Here's how the part is built. I have some questions about the finished solid (model axes, mm). Coordinates: 2 decimals unless noted, no trailing zeros. Order: outer loops, then holes, each group sorted by start corner. A loop starts at its lowest first (then second) coordinate and runs counter-clockwise, first axis right, second up.
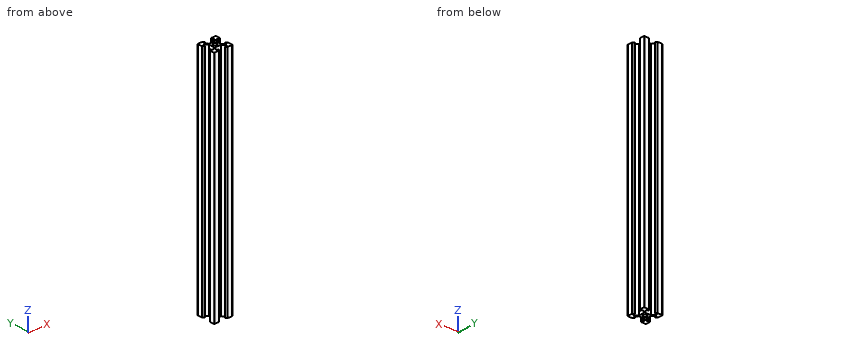
```python
from build123d import *

# Parameters (mm, degrees)
SKETCH1_R           = 2.05
BOSS_EXTRUDE1_DEPTH = 250


with BuildPart() as part:
    # Sketch1 → Boss-Extrude1 (new body)
    with BuildSketch(Plane(origin=(0, 0, 0), x_dir=(0, 1, 0), z_dir=(0, 0, 1))):
        with BuildLine():
            Line((-2.860050506, -3.85), (2.860050506, -3.85))
            Line((2.860050506, -3.85), (5.5, -6.489949494))
            Line((5.5, -6.489949494), (5.5, -8.1))
            Line((5.5, -8.1), (3.382842712, -8.1))
            ThreePointArc((3.382842712, -8.1), (3.198066806, -8.223463314), (3.241421356, -8.441421356))
            Line((3.241421356, -8.441421356), (4.624264069, -9.824264069))
            ThreePointArc((4.624264069, -9.824264069), (4.818918078, -9.95432772), (5.048528137, -10))
            Line((5.048528137, -10), (9.5, -10))
            ThreePointArc((9.5, -10), (9.853553391, -9.853553391), (10, -9.5))
            Line((10, -9.5), (10, -5.048528137))
            ThreePointArc((10, -5.048528137), (9.95432772, -4.818918078), (9.824264069, -4.624264069))
            Line((9.824264069, -4.624264069), (8.441421356, -3.241421356))
            ThreePointArc((8.441421356, -3.241421356), (8.223463314, -3.198066806), (8.1, -3.382842712))
            Line((8.1, -3.382842712), (8.1, -5.5))
            Line((8.1, -5.5), (6.489949494, -5.5))
            Line((6.489949494, -5.5), (3.85, -2.860050506))
            Line((3.85, -2.860050506), (3.85, 2.860050506))
            Line((3.85, 2.860050506), (6.489949494, 5.5))
            Line((6.489949494, 5.5), (8.1, 5.5))
            Line((8.1, 5.5), (8.1, 3.382842712))
            ThreePointArc((8.1, 3.382842712), (8.223463314, 3.198066806), (8.441421356, 3.241421356))
            Line((8.441421356, 3.241421356), (9.824264069, 4.624264069))
            ThreePointArc((9.824264069, 4.624264069), (9.95432772, 4.818918078), (10, 5.048528137))
            Line((10, 5.048528137), (10, 9.5))
            ThreePointArc((10, 9.5), (9.853553391, 9.853553391), (9.5, 10))
            Line((9.5, 10), (5.048528137, 10))
            ThreePointArc((5.048528137, 10), (4.818918078, 9.95432772), (4.624264069, 9.824264069))
            Line((4.624264069, 9.824264069), (3.241421356, 8.441421356))
            ThreePointArc((3.241421356, 8.441421356), (3.198066806, 8.223463314), (3.382842712, 8.1))
            Line((3.382842712, 8.1), (5.5, 8.1))
            Line((5.5, 8.1), (5.5, 6.489949494))
            Line((5.5, 6.489949494), (2.860050506, 3.85))
            Line((2.860050506, 3.85), (-2.860050506, 3.85))
            Line((-2.860050506, 3.85), (-5.5, 6.489949494))
            Line((-5.5, 6.489949494), (-5.5, 8.1))
            Line((-5.5, 8.1), (-3.382842712, 8.1))
            ThreePointArc((-3.382842712, 8.1), (-3.198066806, 8.223463314), (-3.241421356, 8.441421356))
            Line((-3.241421356, 8.441421356), (-4.624264069, 9.824264069))
            ThreePointArc((-4.624264069, 9.824264069), (-4.818918078, 9.95432772), (-5.048528137, 10))
            Line((-5.048528137, 10), (-9.5, 10))
            ThreePointArc((-9.5, 10), (-9.853553391, 9.853553391), (-10, 9.5))
            Line((-10, 9.5), (-10, 5.048528137))
            ThreePointArc((-10, 5.048528137), (-9.95432772, 4.818918078), (-9.824264069, 4.624264069))
            Line((-9.824264069, 4.624264069), (-8.441421356, 3.241421356))
            ThreePointArc((-8.441421356, 3.241421356), (-8.223463314, 3.198066806), (-8.1, 3.382842712))
            Line((-8.1, 3.382842712), (-8.1, 5.5))
            Line((-8.1, 5.5), (-6.489949494, 5.5))
            Line((-6.489949494, 5.5), (-3.85, 2.860050506))
            Line((-3.85, 2.860050506), (-3.85, -2.860050506))
            Line((-3.85, -2.860050506), (-6.489949494, -5.5))
            Line((-6.489949494, -5.5), (-8.1, -5.5))
            Line((-8.1, -5.5), (-8.1, -3.382842712))
            ThreePointArc((-8.1, -3.382842712), (-8.223463314, -3.198066806), (-8.441421356, -3.241421356))
            Line((-8.441421356, -3.241421356), (-9.824264069, -4.624264069))
            ThreePointArc((-9.824264069, -4.624264069), (-9.95432772, -4.818918078), (-10, -5.048528137))
            Line((-10, -5.048528137), (-10, -9.5))
            ThreePointArc((-10, -9.5), (-9.853553391, -9.853553391), (-9.5, -10))
            Line((-9.5, -10), (-5.048528137, -10))
            ThreePointArc((-5.048528137, -10), (-4.818918078, -9.95432772), (-4.624264069, -9.824264069))
            Line((-4.624264069, -9.824264069), (-3.241421356, -8.441421356))
            ThreePointArc((-3.241421356, -8.441421356), (-3.198066806, -8.223463314), (-3.382842712, -8.1))
            Line((-3.382842712, -8.1), (-5.5, -8.1))
            Line((-5.5, -8.1), (-5.5, -6.489949494))
            Line((-5.5, -6.489949494), (-2.860050506, -3.85))
        make_face()
        with Locations(Location((0, 0, 0), (0, 0, 270))):
            Circle(SKETCH1_R, mode=Mode.SUBTRACT)
    extrude(amount=BOSS_EXTRUDE1_DEPTH)


solid = part.part
```
Q1. Will these pins go through, and if not, where does the flat tip stop? pin 1 (8 mm diameter, centred on x = 1, z = 134.5, fed in from -Y); pin 2 (6.5 mm diameter, centred on y = 1.5, z = 129, fed in from -X); pin 3 (0.6 mm diameter, centred on y = 4, z = 113, fed in from -X); pin 4 (1.5 mm diameter, centred on x = -1, y = 6, fed in from +Z).
Q2. If we section it at A-A on x = 0: Write out the boundary of the cut face in (y, z), then the cut area to 3 significant figures.
Q3. I need wall thicknesses on L1, parallel to X at y = 7, z = 58.5; L2, parallel to Y at x = 0, z = 196.5. Which ranges of each line are inside material? Lowest first, please.
Reply:
1. pin 1: stops at y = -10
1. pin 2: stops at x = -9.92
1. pin 3: stops at x = -9.5
1. pin 4: passes through
2. outline: (-3.85, 0) - (-2.05, 0) - (-2.05, 250) - (-3.85, 250) - close; (2.05, 0) - (3.85, 0) - (3.85, 250) - (2.05, 250) - close
2. area: 900 mm2
3. L1: x = -10 to -5.5, 5.5 to 10
3. L2: y = -3.85 to -2.05, 2.05 to 3.85
